from build123d import *

# Parameters (mm, degrees)
SKETCH1_R               = 100
BOSS_EXTRUDE3_DEPTH     = 90
SKETCH4_W               = 40
SKETCH4_H               = 60
CUT_EXTRUDE2_DEPTH      = 26
CUT_EXTRUDE2_DEPTH_BACK = 12
SKETCH12_R              = 100
BOSS_EXTRUDE4_DEPTH     = 0.1
SKETCH13_R              = 86
CUT_EXTRUDE8_DEPTH      = 80
SKETCH18_R              = 32.5
BOSS_EXTRUDE5_DEPTH     = 25
SKETCH16_R              = 1.6
CUT_EXTRUDE11_DEPTH     = 91.1
SKETCH17_R              = 3
CUT_EXTRUDE12_DEPTH     = 30
SKETCH19_R              = 30
CUT_EXTRUDE13_DEPTH     = 25
SKETCH20_W              = 40
SKETCH20_H              = 5
CUT_EXTRUDE14_DEPTH     = 25
SKETCH21_R              = 1.55
CUT_EXTRUDE15_DEPTH     = 25
CUT_EXTRUDE16_DEPTH     = 35
SKETCH23_W              = 30
SKETCH23_H              = 15
CUT_EXTRUDE17_DEPTH     = 20


with BuildPart() as part:
    # Sketch1 → Boss-Extrude3 (new body)
    with BuildSketch(Plane(origin=(0, 0, 0), x_dir=(1, 0, 0), z_dir=(0, 1, 0))):
        Circle(SKETCH1_R)
    extrude(amount=BOSS_EXTRUDE3_DEPTH)

    # Sketch4 → Cut-Extrude2 (cut, two sides)
    with BuildSketch(Plane.XY.offset(105)) as cut_extrude2_sk:
        with Locations((0, 45)):
            Rectangle(SKETCH4_W, SKETCH4_H)
    extrude(amount=CUT_EXTRUDE2_DEPTH, mode=Mode.SUBTRACT)
    extrude(cut_extrude2_sk.sketch, amount=-CUT_EXTRUDE2_DEPTH_BACK, mode=Mode.SUBTRACT)

    # Sketch12 → Boss-Extrude4 (add)
    with BuildSketch(Plane.XZ):
        Circle(SKETCH12_R)
    extrude(amount=BOSS_EXTRUDE4_DEPTH)

    # Sketch13 → Cut-Extrude8 (cut)
    with BuildSketch(Plane(origin=(0, 90, 0), x_dir=(1, 0, 0), z_dir=(0, 1, 0))):
        Circle(SKETCH13_R)
    extrude(amount=-CUT_EXTRUDE8_DEPTH, mode=Mode.SUBTRACT)

    # Sketch18 → Boss-Extrude5 (add)
    with BuildSketch(Plane(origin=(0, 10, 0), x_dir=(1, 0, 0), z_dir=(0, 1, 0))):
        Circle(SKETCH18_R)
    extrude(amount=BOSS_EXTRUDE5_DEPTH)

    # Sketch16 → Cut-Extrude11 (cut, through all)
    with BuildSketch(Plane.XZ.offset(0.1)):
        with Locations((-15, 15.5)):
            Circle(SKETCH16_R)
        with Locations((15, 15.5)):
            Circle(SKETCH16_R)
        with Locations((15, -15.5)):
            Circle(SKETCH16_R)
        with Locations((-15, -15.5)):
            Circle(SKETCH16_R)
    extrude(amount=-CUT_EXTRUDE11_DEPTH, mode=Mode.SUBTRACT)

    # Sketch17 → Cut-Extrude12 (cut)
    with BuildSketch(Plane.XZ.offset(0.1)):
        with Locations((-15, 15.5)):
            Circle(SKETCH17_R)
        with Locations((15, 15.5)):
            Circle(SKETCH17_R)
        with Locations((-15, -15.5)):
            Circle(SKETCH17_R)
        with Locations((15, -15.5)):
            Circle(SKETCH17_R)
    extrude(amount=-CUT_EXTRUDE12_DEPTH, mode=Mode.SUBTRACT)

    # Sketch19 → Cut-Extrude13 (cut)
    with BuildSketch(Plane.XZ.offset(0.1)):
        Circle(SKETCH19_R)
    extrude(amount=-CUT_EXTRUDE13_DEPTH, mode=Mode.SUBTRACT)

    # Sketch20 → Cut-Extrude14 (cut)
    with BuildSketch(Plane.XY.offset(93)):
        with Locations((0, 17.5)):
            Rectangle(SKETCH20_W, SKETCH20_H)
    extrude(amount=-CUT_EXTRUDE14_DEPTH, mode=Mode.SUBTRACT)

    # Sketch21 → Cut-Extrude15 (cut)
    with BuildSketch(Plane.XY.offset(93)):
        with Locations((12.45, 67.8)):
            Circle(SKETCH21_R)
        with Locations((-12.45, 67.8)):
            Circle(SKETCH21_R)
        with Locations((-17.05, 30.54)):
            Circle(SKETCH21_R)
        with Locations((17.05, 30.54)):
            Circle(SKETCH21_R)
    extrude(amount=-CUT_EXTRUDE15_DEPTH, mode=Mode.SUBTRACT)

    # Sketch22 → Cut-Extrude16 (cut)
    with BuildSketch(Plane(origin=(22.204096953, 47.794122581, -296.404157649), x_dir=(1, 0, 0), z_dir=(0, 1, 0))):
        Polygon((-6.791929493, -346.959107226), (12.404969277, -405.762485644), (37.058002756, -394.3841625), (3.953655983, -342.212063172), align=None)
    extrude(amount=CUT_EXTRUDE16_DEPTH, mode=Mode.SUBTRACT)

    # Sketch23 → Cut-Extrude17 (cut)
    with BuildSketch(Plane.XY.offset(-100)):
        with Locations((-0.77861777, 17.5)):
            Rectangle(SKETCH23_W, SKETCH23_H)
    extrude(amount=CUT_EXTRUDE17_DEPTH, mode=Mode.SUBTRACT)


solid = part.part
Part model, mm, in its own coordinate system. A direction names the side the tool comes from. Give positions to 0.01 mm unless a question says otherwise; leave off trailing zeros. Order: outer loops, then holes, each group sorted by start corner. A loop starts at its lowest first (then second) coordinate and runs counter-clockwise, first axis right, second up. Notation, with made-up numbers: (65, -15.75) - (72, -15.75) arc R18 cw to (72, -10.75) - close; hole circle Ø3 at (-1, -24). An arc over 180 degrees is marked (long way). Use a Markdown table: item, result.
1) 3-axis set-ups, long thin cutter, end or side, ignore diameter. For faces 1 (the flat face through (27.843, 65.049, 88.632)), 2 (the flat face through (14.221, 17, -92)), 3 (the flat face through (0, 75, 97)), 4 (the flat face through (-14, 29.9, -17)), 5 (the cylindrical face through (31, 22.32, -9.76)): which of +Z, -Z, +X, -X, +Y, -Y reach the whole face in a straight line?
Checked values:
| item | result |
|---|---|
| face 1 | none |
| face 2 | -Z |
| face 3 | +Z |
| face 4 | -Y |
| face 5 | +Y |
2) Two-plate mould, pull along Z, no slides. Class faces 6 (the flat face through (0, 48, 93)), 7 (the cylindrical face through (-63.39, 50.56, -58.12)), 8 (the flat face through (-20, 38, 94)): +Z half, -Z half, draft (parallel to the pull), parting line (faces both ways), or undercut.
Checked values:
| item | result |
|---|---|
| face 6 | +Z half |
| face 7 | undercut |
| face 8 | draft |
3) Saw through at B-B on z = 0. List the corners of the cut face in (x, y), plus the area to 4 significant figures.
Checked values:
| item | result |
|---|---|
| outline | (-100, -0.1) - (-30, -0.1) - (-30, 24.9) - (30, 24.9) - (30, -0.1) - (100, -0.1) - (100, 90) - (86, 90) - (86, 10) - (32.5, 10) - (32.5, 35) - (-32.5, 35) - (-32.5, 10) - (-86, 10) - (-86, 90) - (-100, 90) - close |
| area | 4,385 mm² |
4) Saw through at D-D on x = 69. List the corners of the cut face in (y, z).
Checked values:
| item | result |
|---|---|
| outline | (-0.1, -72.38) - (90, -72.38) - (90, -51.33) - (10, -51.33) - (10, 51.33) - (90, 51.33) - (90, 72.38) - (-0.1, 72.38) - close |
5) Saw through at A-A on x = 0. List the corners of the cut face in (y, z).
Checked values:
| item | result |
|---|---|
| outline | (-0.1, -100) - (10, -100) - (10, -32.5) - (35, -32.5) - (35, 32.5) - (10, 32.5) - (10, 86) - (15, 86) - (15, 100) - (-0.1, 100) - (-0.1, 30) - (24.9, 30) - (24.9, -30) - (-0.1, -30) - close; (20, 86) - (90, 86) - (90, 100) - (75, 100) - (75, 93) - (20, 93) - close; (25, -100) - (90, -100) - (90, -86) - (25, -86) - close |
6) Flat gauge pins, fed straight in: P1, Ø15.5, axis at y = 16.5, z = -91.5, coming from the -X side; P2, Ø5, axis at x = -17.05, y = 30.54, coming from the +Z side; P3, Ø2, axis at x = 34.5, y = 69.5, coming from the +Z side. Where does each tip first touch, or does it go through?
Checked values:
| item | result |
|---|---|
| P1 | x = -54.64 |
| P2 | z = 93 |
| P3 | z = -78.33 |
7) Saw through at C-C on y = 53.5. List the corners of the cut face in (x, z).
Checked values:
| item | result |
|---|---|
| outline | (-20, 93) - (-20, 97.98) arc R100 ccw (long way) to (51.49, 85.73) - (43.98, 73.9) arc R86 cw (long way) to (25.7, 82.07) - (30.05, 95.38) arc R100 ccw to (20, 97.98) - (20, 93) - close |
8) Probe L1, parallel to X at y = 67.8, z = 86.5; L2, parallel to X at y = 53, z = 0; L3, parallel to X at y = 54, z = -3. List the from-to ranges inside material, lowest first. Write a range as from..to.
Checked values:
| item | result |
|---|---|
| L1 | -50.18..-14, -10.9..10.9, 14..27.15 |
| L2 | -100..-86, 86..100 |
| L3 | -99.95..-85.95, 85.95..99.95 |
